from build123d import *

# Parameters (mm, degrees)
BOSS_EXTRUDE2_DEPTH                               = 22.225
BOSS_EXTRUDE2_DEPTH_BACK                          = 10
SKETCH2_W                                         = 153.14353988
SKETCH2_H                                         = 6.35
CUT_EXTRUDE1_DEPTH                                = 4.7625
SKETCH3_W                                         = 152.758434582
SKETCH3_H                                         = 6.35
CUT_EXTRUDE2_DEPTH                                = 4.7625
FILLET3_R                                         = 12.7
FILLET4_R                                         = 12.7
FILLET5_R                                         = 12.7
FILLET6_R                                         = 12.7
CUT_EXTRUDE3_DEPTH                                = 94.675
CUT_EXTRUDE3_DEPTH_BACK                           = 84.675
SKETCH12_R                                        = 168.402
CSK_FOR_8_FLAT_HEAD_SOCKET_CAP_SCREW2_D           = 4.4958
CSK_FOR_8_FLAT_HEAD_SOCKET_CAP_SCREW2_CSINK_D     = 9.1186
CSK_FOR_8_FLAT_HEAD_SOCKET_CAP_SCREW2_CSINK_ANGLE = 82
SKETCH22_W                                        = 144.636542349
SKETCH22_H                                        = 24.041785527
CUT_EXTRUDE4_DEPTH                                = 42.672


with BuildPart() as part:
    # Sketch1 → Boss-Extrude2 (new, two sides: drawn at the far end of the back side and taken through both)
    with BuildSketch(Plane(origin=(0, 0, 0), x_dir=(1, 0, 0), z_dir=(0, 1, 0)).offset(-BOSS_EXTRUDE2_DEPTH_BACK)):
        with BuildLine():
            Line((37.204956004, 9.525), (-37.204956004, 9.525))
            ThreePointArc((-37.204956004, 9.525), (-39.498289417, 9.316221792), (-41.716221563, 8.696751473))
            Line((-41.716221563, 8.696751473), (-62.649818949, 0.741984467))
            ThreePointArc((-62.649818949, 0.741984467), (-63.161614851, 0), (-62.649818949, -0.741984467))
            Line((-62.649818949, -0.741984467), (-41.716221563, -8.696751473))
            ThreePointArc((-41.716221563, -8.696751473), (-39.498289417, -9.316221792), (-37.204956004, -9.525))
            Line((-37.204956004, -9.525), (37.204956004, -9.525))
            ThreePointArc((37.204956004, -9.525), (39.498289417, -9.316221792), (41.716221563, -8.696751473))
            Line((41.716221563, -8.696751473), (62.649818949, -0.741984467))
            ThreePointArc((62.649818949, -0.741984467), (63.161614851, 0), (62.649818949, 0.741984467))
            Line((62.649818949, 0.741984467), (41.716221563, 8.696751473))
            ThreePointArc((41.716221563, 8.696751473), (39.498289417, 9.316221792), (37.204956004, 9.525))
        make_face()
    extrude(amount=BOSS_EXTRUDE2_DEPTH + BOSS_EXTRUDE2_DEPTH_BACK)

    # Sketch2 → Cut-Extrude1 (cut)
    with BuildSketch(Plane.XY.offset(9.525)):
        with Locations((7.894658594, 12.7)):
            Rectangle(SKETCH2_W, SKETCH2_H)
    extrude(amount=-CUT_EXTRUDE1_DEPTH, mode=Mode.SUBTRACT)

    # Sketch3 → Cut-Extrude2 (cut)
    with BuildSketch(Plane(origin=(0, 0, -9.525), x_dir=(-1, 0, 0), z_dir=(0, 0, -1))):
        with Locations((8.600684972, 12.7)):
            Rectangle(SKETCH3_W, SKETCH3_H)
    extrude(amount=-CUT_EXTRUDE2_DEPTH, mode=Mode.SUBTRACT)

    # Fillet3
    fillet3_edges = [part.edges().sort_by_distance(p)[0] for p in [
        (52.069514915, 12.7, -4.7625),
    ]]
    fillet(fillet3_edges, radius=FILLET3_R)

    # Fillet4
    fillet4_edges = [part.edges().sort_by_distance(p)[0] for p in [
        (52.069514915, 12.7, 4.7625),
    ]]
    fillet(fillet4_edges, radius=FILLET4_R)

    # Fillet5
    fillet5_edges = [part.edges().sort_by_distance(p)[0] for p in [
        (-52.069514915, 12.7, 4.7625),
    ]]
    fillet(fillet5_edges, radius=FILLET5_R)

    # Fillet6
    fillet6_edges = [part.edges().sort_by_distance(p)[0] for p in [
        (-52.069514915, 12.7, -4.7625),
    ]]
    fillet(fillet6_edges, radius=FILLET6_R)

    # Sketch12 → Cut-Extrude3 (cut, two sides: drawn at the far end of the back side and taken through both)
    with BuildSketch(Plane(origin=(0, 0, 0), x_dir=(0, 0, -1), z_dir=(1, 0, 0)).offset(-CUT_EXTRUDE3_DEPTH_BACK)):
        with Locations((0, -168.402)):
            Circle(SKETCH12_R)
    extrude(amount=CUT_EXTRUDE3_DEPTH + CUT_EXTRUDE3_DEPTH_BACK, mode=Mode.SUBTRACT)

    # CSK for #8 Flat Head Socket Cap Screw2 (through all)
    with Locations(Plane(origin=(0, 22.225, 0), x_dir=(1, 0, 0), z_dir=(0, 1, 0))):
        with Locations((-44.45, 0), (44.45, 0)):
            CounterSinkHole(CSK_FOR_8_FLAT_HEAD_SOCKET_CAP_SCREW2_D / 2, CSK_FOR_8_FLAT_HEAD_SOCKET_CAP_SCREW2_CSINK_D / 2, counter_sink_angle=CSK_FOR_8_FLAT_HEAD_SOCKET_CAP_SCREW2_CSINK_ANGLE)

    # Sketch22 → Cut-Extrude4 (cut)
    with BuildSketch(Plane(origin=(0, 3.175, 0), x_dir=(1, 0, 0), z_dir=(0, 1, 0))):
        with Locations((-1.245916594, -0.077514015)):
            Rectangle(SKETCH22_W, SKETCH22_H)
    extrude(amount=CUT_EXTRUDE4_DEPTH, mode=Mode.SUBTRACT)


solid = part.part
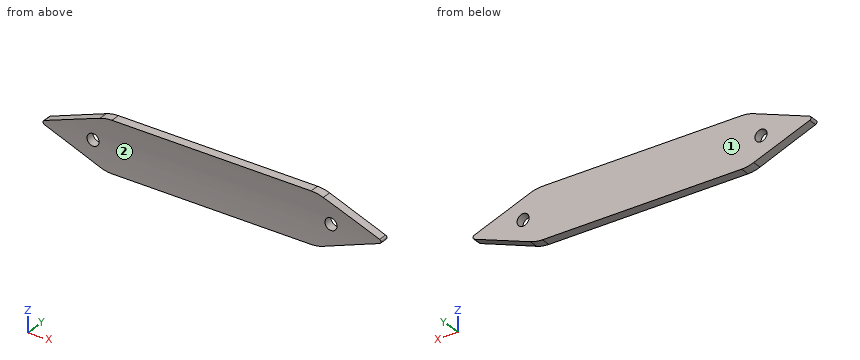
Geometry: final body of the model. Coordinates: model frame, mm. Face numbers are marked on the shaded views. Give positions to 0.01 mm unless a question says otherwise; leave off trailing zeros. Order: outer loops, then holes, each group sorted by start corner. A loop starts at its lowest first (then second) coordinate and runs counter-clockwise, first axis right, second up. Notation, with made-up numbers: (45, 39) -> (98, 39) arc R12 ccw to (98, 51) -> close; hole circle Ø7 at (80.25, -11). An arc over 180 degrees is marked (long way). Answer as a JSON object with one key per item and string values.
Q1. Material intervals for probe 1 along Y at (x, z) = (-9.5, 0.75) (3 decimals); probe 2 along Z at (x, y) = (-44.45, 2.5); probe 3 along Y at (x, z) = (28.5, 8.75) (3 decimals), sorted ascending.
Entries:
{"probe 1": "y = -0.002 to 3.175", "probe 2": "z = -7.66 to -2.25, 2.25 to 7.66", "probe 3": "y = -0.227 to 3.175"}
Q2. Section C-C (x = 30.5). Output: boundary loops of the cut face in (y, z) (3 decimals).
Entries:
{"outline": "(-0.27, -9.525) -> (3.175, -9.525) -> (3.175, 9.525) -> (-0.27, 9.525) arc R168.402 cw to start"}
Q3. Section A-A (y = 1.6). State how many separate pieces and enclosed holes the cut face has, plus the area to 3 significant figures.
Entries:
{"separate pieces": "1", "enclosed holes": "2", "area": "1,950 mm^2"}
Q4. Section B-B (x = -44.45). Output: boundary loops of the cut face in (y, z) (3 decimals).
Entries:
{"outline": "(-0.174, -7.658) -> (3.175, -7.658) -> (3.175, -2.248) -> (-0.015, -2.248) arc R168.402 cw to start; (-0.174, 7.658) arc R168.402 cw to (-0.015, 2.248) -> (3.175, 2.248) -> (3.175, 7.658) -> close"}
Q5. Section D-D (z = 6.75). Output: boundary loops of the cut face in (x, y) (3 decimals), plus the area to 3 significant figures.
Entries:
{"outline": "(-46.839, -0.135) -> (46.839, -0.135) -> (46.839, 3.175) -> (-46.839, 3.175) -> close", "area": "310 mm^2"}
Q6. First-contact query: pin 1 (5 mm diameter, centred on x = -38.5, z = 1.5, fed in from -Y); pin 2 (7 mm diameter, centred on x = 44.45, z = 0, fed in from +Y) (3 decimals). Flat tips, straight axial feed; report the tip coordinate or a pass-through.
Entries:
{"pin 1": "stops at y = -0.05", "pin 2": "stops at y = 3.175"}
Q7. Draft query along Z for the marked faces 1 and 2. Return one class per face: released by +Z, released by -Z, zero draft, split by the parting line, or undercut.
Entries:
{"face 1": "zero draft", "face 2": "undercut"}
